from build123d import *

# Parameters (mm, degrees)
BOSS_EXTRUDE1_DEPTH  = 203.2
SKETCH2_R            = 2.286
BOSS_EXTRUDE2_DEPTH  = 6.35
FILLET1_R            = 2.54
FILLET1_OF_MIRROR1_R = 2.54
SKETCH5_W            = 6.35
SKETCH5_H            = 9.597846327
CUT_EXTRUDE3_DEPTH   = 207.350575478
SKETCH3_W            = 6.277153673
SKETCH3_H            = 3.048
CUT_EXTRUDE1_DEPTH   = 205.701857736
SKETCH4_W            = 4.826
SKETCH4_H            = 3.175
CUT_EXTRUDE2_DEPTH   = 206.39013623
CHAMFER1_SIZE        = 0.762


with BuildPart() as part:
    # Sketch1 → Boss-Extrude1 (new body)
    with BuildSketch(Plane(origin=(0, 0, 0), x_dir=(1, 0, 0), z_dir=(0, 1, 0))):
        Polygon((0, 0), (25.4, 0), (25.4, 25.4), (19.05, 25.4), (19.05, 6.35), (0, 6.35), align=None)
    extrude(amount=BOSS_EXTRUDE1_DEPTH)

    # Sketch2 → Boss-Extrude2 (add)
    with BuildSketch(Plane(origin=(0, 203.2, 0), x_dir=(1, 0, 0), z_dir=(0, 1, 0))):
        with BuildLine():
            Line((19.05, 15.802153673), (19.05, 6.35))
            Line((19.05, 6.35), (8.89, 6.35))
            Line((8.89, 6.35), (9.629456844, 12.244049961))
            ThreePointArc((9.629456844, 12.244049961), (10.972967985, 14.785452355), (13.661846327, 15.802153673))
            Line((13.661846327, 15.802153673), (19.05, 15.802153673))
        make_face()
        with Locations(Location((13.661846327, 11.738153673, 0), (0, 0, 270))):
            Circle(SKETCH2_R, mode=Mode.SUBTRACT)
    boss_extrude2 = extrude(amount=-BOSS_EXTRUDE2_DEPTH)

    # Fillet1
    fillet1_edges = [part.edges().sort_by_distance(p)[0] for p in [
        (8.89, 200.025, -6.35),
    ]]
    fillet(fillet1_edges, radius=FILLET1_R)

    # Mirror1: Boss-Extrude2 across plane
    add(boss_extrude2.mirror(Plane.ZX.offset(101.6)))

    # Fillet1 of Mirror1
    fillet1_of_mirror1_edges = [part.edges().sort_by_distance(p)[0] for p in [
        (8.89, 3.175, -6.35),
    ]]
    fillet(fillet1_of_mirror1_edges, radius=FILLET1_OF_MIRROR1_R)

    # Sketch5 → Cut-Extrude3 (cut, through all)
    with BuildSketch(Plane(origin=(0, 203.2, 0), x_dir=(1, 0, 0), z_dir=(0, 1, 0))):
        with Locations((22.225, 20.601076837)):
            Rectangle(SKETCH5_W, SKETCH5_H)
    extrude(amount=-CUT_EXTRUDE3_DEPTH, mode=Mode.SUBTRACT)

    # Sketch3 → Cut-Extrude1 (cut, through all)
    with BuildSketch(Plane.ZY.offset(-19.05)):
        with Locations((-12.663576837, 188.976)):
            Rectangle(SKETCH3_W, SKETCH3_H)
        with Locations((-12.663576837, 182.950068966)):
            Rectangle(SKETCH3_W, SKETCH3_H)
        with Locations((-12.663576837, 176.924137931)):
            Rectangle(SKETCH3_W, SKETCH3_H)
        with Locations((-12.663576837, 170.898206897)):
            Rectangle(SKETCH3_W, SKETCH3_H)
        with Locations((-12.663576837, 164.872275862)):
            Rectangle(SKETCH3_W, SKETCH3_H)
        with Locations((-12.663576837, 158.846344828)):
            Rectangle(SKETCH3_W, SKETCH3_H)
        with Locations((-12.663576837, 152.820413793)):
            Rectangle(SKETCH3_W, SKETCH3_H)
        with Locations((-12.663576837, 146.794482759)):
            Rectangle(SKETCH3_W, SKETCH3_H)
        with Locations((-12.663576837, 140.768551724)):
            Rectangle(SKETCH3_W, SKETCH3_H)
        with Locations((-12.663576837, 134.74262069)):
            Rectangle(SKETCH3_W, SKETCH3_H)
        with Locations((-12.663576837, 128.716689655)):
            Rectangle(SKETCH3_W, SKETCH3_H)
        with Locations((-12.663576837, 122.690758621)):
            Rectangle(SKETCH3_W, SKETCH3_H)
        with Locations((-12.663576837, 116.664827586)):
            Rectangle(SKETCH3_W, SKETCH3_H)
        with Locations((-12.663576837, 110.638896552)):
            Rectangle(SKETCH3_W, SKETCH3_H)
        with Locations((-12.663576837, 104.612965517)):
            Rectangle(SKETCH3_W, SKETCH3_H)
        with Locations((-12.663576837, 98.587034483)):
            Rectangle(SKETCH3_W, SKETCH3_H)
        with Locations((-12.663576837, 92.561103448)):
            Rectangle(SKETCH3_W, SKETCH3_H)
        with Locations((-12.663576837, 86.535172414)):
            Rectangle(SKETCH3_W, SKETCH3_H)
        with Locations((-12.663576837, 80.509241379)):
            Rectangle(SKETCH3_W, SKETCH3_H)
        with Locations((-12.663576837, 74.483310345)):
            Rectangle(SKETCH3_W, SKETCH3_H)
        with Locations((-12.663576837, 68.45737931)):
            Rectangle(SKETCH3_W, SKETCH3_H)
        with Locations((-12.663576837, 62.431448276)):
            Rectangle(SKETCH3_W, SKETCH3_H)
        with Locations((-12.663576837, 56.405517241)):
            Rectangle(SKETCH3_W, SKETCH3_H)
        with Locations((-12.663576837, 50.379586207)):
            Rectangle(SKETCH3_W, SKETCH3_H)
        with Locations((-12.663576837, 44.353655172)):
            Rectangle(SKETCH3_W, SKETCH3_H)
        with Locations((-12.663576837, 38.327724138)):
            Rectangle(SKETCH3_W, SKETCH3_H)
        with Locations((-12.663576837, 32.301793103)):
            Rectangle(SKETCH3_W, SKETCH3_H)
        with Locations((-12.663576837, 26.275862069)):
            Rectangle(SKETCH3_W, SKETCH3_H)
        with Locations((-12.663576837, 20.249931034)):
            Rectangle(SKETCH3_W, SKETCH3_H)
        with Locations((-12.663576837, 14.224)):
            Rectangle(SKETCH3_W, SKETCH3_H)
    extrude(amount=-CUT_EXTRUDE1_DEPTH, mode=Mode.SUBTRACT)

    # Sketch4 → Cut-Extrude2 (cut, through all)
    with BuildSketch(Plane.XZ):
        with Locations((2.413, -3.175)):
            Rectangle(SKETCH4_W, SKETCH4_H)
    extrude(amount=-CUT_EXTRUDE2_DEPTH, mode=Mode.SUBTRACT)

    # Chamfer1
    chamfer1_edges = [part.edges().sort_by_distance(p)[0] for p in [
        (25.4, 161.859310345, -15.802153673),
        (25.4, 167.885241379, -15.802153673),
        (25.4, 173.911172414, -15.802153673),
        (25.4, 179.937103448, -15.802153673),
        (25.4, 185.963034483, -15.802153673),
        (19.05, 161.859310345, -15.802153673),
        (19.05, 167.885241379, -15.802153673),
        (19.05, 173.911172414, -15.802153673),
        (19.05, 179.937103448, -15.802153673),
        (19.05, 185.963034483, -15.802153673),
        (22.225, 187.452, -15.802153673),
        (22.225, 160.370344828, -15.802153673),
        (22.225, 166.396275862, -15.802153673),
        (22.225, 163.348275862, -15.802153673),
        (22.225, 184.474068966, -15.802153673),
        (22.225, 181.426068966, -15.802153673),
        (22.225, 178.448137931, -15.802153673),
        (22.225, 175.400137931, -15.802153673),
        (22.225, 172.422206897, -15.802153673),
        (22.225, 169.374206897, -15.802153673),
    ]]
    chamfer(chamfer1_edges, length=CHAMFER1_SIZE)


solid = part.part
The listing builds one solid part. Answer for the finished solid, in the listing's coordinates (mm). A direction names the side the tool comes from. Round coordinates to 2 decimals unless told otherwise and drop trailing zeros. Loops run counter-clockwise (first coordinate to the right, second up) from the corner with the lowest first, then second, coordinate; pieces in that order, holes last. Notation, with made-up numbers: M -16,6 L 39,6 A38 cw 39,45 Z; hole C 65,-29 d2. An arc over 180 degrees is marked long. Return JSON: item names as keys, results as strings.
Q1. Find section A-A, the plane x = 3. Determine the outline of the cut face in (y, z).
Results list:
{"outline": "M 0,-6.35 L 203.2,-6.35 L 203.2,-4.76 L 0,-4.76 Z; M 0,-1.59 L 203.2,-1.59 L 203.2,0 L 0,0 Z"}
Q2. Which of the six approach directions +Z, -Z, +X, -X, +Y, -Y give full straight-line access (tool end or side, diameter ignored) to faces 1 (the face through (22, 54.882, -13)), 2 (the face through (21, 198, -15.802))?
Results list:
{"face 1": "-Z, +X, -X", "face 2": "-Z, +X, -X, +Y, -Y"}
Q3. Find the intervals of material crossed by line 1 along Y through (x, z) = (10.25, -7.5); line 2 along X through (y, z) = (106.5, -3); line 3 along Z through (x, y) = (14.25, 82), in increasing order. Write a range as from..to.
Results list:
{"line 1": "y = 0..6.35, 196.85..203.2", "line 2": "x = 4.83..25.4", "line 3": "z = -6.35..0"}
Q4. Each of these flat-tipped pins is pushed along its axis until it touches: pin 1 Ø6 at (x, y) = (7, 113.5) entering from -Z; pin 2 Ø2.5 at (x, y) = (22.5, 74.5) entering from -Z (3 decimals); pin 3 Ø3.5 at (x, z) = (13.66, -11.74) entering from -Y. Where does it stop, or does it pass through?
Results list:
{"pin 1": "stops at z = -6.35", "pin 2": "stops at z = -9.525", "pin 3": "passes through"}
Q5. The mould has two halves that part along Y. Classify faces 3 (the face through (22, 97.063, -13)), 4 (the face through (16, 0, -6)), 5 (the face through (15.59, 3.13, -10.51)): released by +Y, released by -Y, zero draft, split by the parting line, or undercut.
Results list:
{"face 3": "undercut", "face 4": "released by -Y", "face 5": "zero draft"}
